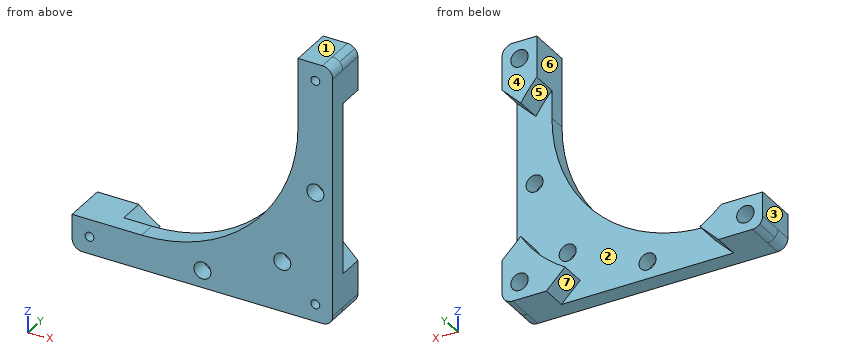
```python
from build123d import *

# Parameters (mm, degrees)
SKETCH1_W               = 190.5
SKETCH1_H               = 190.5
BOSS_EXTRUDE1_DEPTH     = 12.7
FILLET1_R               = 7.62
BOSS_EXTRUDE3_START     = 19.05
BOSS_EXTRUDE3_DEPTH     = 19.05
CIRPATTERN1_COUNT       = 4
SKETCH8_R               = 6.223
CUT_EXTRUDE2_DEPTH      = 25.4
CUT_EXTRUDE3_DEPTH      = 137.044211564
CUT_EXTRUDE3_DEPTH_BACK = 137.044211564
SKETCH10_R              = 6.223
FILLET2_R               = 12.7
SKETCH11_R              = 6.35
CUT_EXTRUDE4_DEPTH      = 19.05
SKETCH11_3_R            = 3.2385
CUT_EXTRUDE5_DEPTH      = 139.395041457
CIRPATTERN2_COUNT       = 4
CUT_EXTRUDE6_DEPTH      = 137.044211564
CUT_EXTRUDE6_DEPTH_BACK = 137.044211564
CUT_EXTRUDE7_DEPTH      = 137.044211564
CUT_EXTRUDE7_DEPTH_BACK = 137.044211564


with BuildPart() as part:
    # Sketch1 → Boss-Extrude1 (new body)
    with BuildSketch(Plane(origin=(0, 0, 0), x_dir=(1, 0, 0), z_dir=(0, 1, 0))):
        Rectangle(SKETCH1_W, SKETCH1_H)
    extrude(amount=BOSS_EXTRUDE1_DEPTH)

    # Fillet1
    fillet1_edges = [part.edges().sort_by_distance(p)[0] for p in [
        (95.25, 6.35, 95.25),
        (-95.25, 6.35, 95.25),
        (-95.25, 6.35, -95.25),
        (95.25, 6.35, -95.25),
    ]]
    fillet(fillet1_edges, radius=FILLET1_R)

    # Sketch7 → Boss-Extrude3 (add)
    with BuildSketch(Plane(origin=(0, 12.7, 0), x_dir=(1, 0, 0), z_dir=(0, 1, 0)).offset(BOSS_EXTRUDE3_START)):
        with BuildLine():
            Line((67.396822189, 67.396822189), (93.018153673, 93.018153673))
            ThreePointArc((93.018153673, 93.018153673), (90.546047755, 94.669962038), (87.63, 95.25))
            Line((87.63, 95.25), (62.921077964, 95.25))
            Line((62.921077964, 95.25), (49.265209936, 81.594131972))
            ThreePointArc((49.265209936, 81.594131972), (58.761367718, 75.045086089), (67.396822189, 67.396822189))
        make_face()
        with BuildLine():
            ThreePointArc((95.25, 87.63), (94.669962038, 90.546047755), (93.018153673, 93.018153673))
            Line((93.018153673, 93.018153673), (67.396822189, 67.396822189))
            ThreePointArc((67.396822189, 67.396822189), (75.045086089, 58.761367718), (81.594131972, 49.265209936))
            Line((81.594131972, 49.265209936), (95.25, 62.921077964))
            Line((95.25, 62.921077964), (95.25, 87.63))
        make_face()
    boss_extrude3 = extrude(amount=-BOSS_EXTRUDE3_DEPTH)

    # CirPattern1: Boss-Extrude3 ×4 about axis
    cirpattern1_axis = Axis((0, 0, 0), (0, 1, 0))
    for i in range(1, CIRPATTERN1_COUNT):
        add(boss_extrude3.rotate(cirpattern1_axis, i * 360 / CIRPATTERN1_COUNT))

    # Sketch8 → Cut-Extrude2 (cut)
    with BuildSketch(Plane(origin=(0, 12.7, 0), x_dir=(1, 0, 0), z_dir=(0, 1, 0))):
        with Locations(Location((0, 82.55, 0), (0, 0, 270))):
            Circle(SKETCH8_R)
        with Locations(Location((58.371664787, 58.371664787, 0), (0, 0, 270))):
            Circle(SKETCH8_R)
        with Locations(Location((82.55, 0, 0), (0, 0, 270))):
            Circle(SKETCH8_R)
        with Locations(Location((58.371664787, -58.371664787, 0), (0, 0, 270))):
            Circle(SKETCH8_R)
        with Locations(Location((0, -82.55, 0), (0, 0, 270))):
            Circle(SKETCH8_R)
        with Locations(Location((-58.371664787, -58.371664787, 0), (0, 0, 270))):
            Circle(SKETCH8_R)
        with Locations(Location((-82.55, 0, 0), (0, 0, 270))):
            Circle(SKETCH8_R)
        with Locations(Location((-58.371664787, 58.371664787, 0), (0, 0, 270))):
            Circle(SKETCH8_R)
    extrude(amount=-CUT_EXTRUDE2_DEPTH, mode=Mode.SUBTRACT)

    # Sketch10 → Cut-Extrude3 (cut, two sides: drawn at the far end of the back side and taken through both)
    # profile 1 of 2: a face of its own
    with BuildSketch(Plane(origin=(0, 12.7, 0), x_dir=(1, 0, 0), z_dir=(0, 1, 0)).offset(-CUT_EXTRUDE3_DEPTH_BACK)):
        Polygon((38.1, 38.1), (-95.25, 38.1), (-95.25, -38.1), (-38.1, -38.1), (-38.1, -95.25), (38.1, -95.25), align=None)
        with Locations((-82.55, 0)):
            Circle(SKETCH10_R, mode=Mode.SUBTRACT)
        with Locations((0, -82.55)):
            Circle(SKETCH10_R, mode=Mode.SUBTRACT)
    # profile 2 of 2: a face of its own
    with BuildSketch(Plane(origin=(0, 12.7, 0), x_dir=(1, 0, 0), z_dir=(0, 1, 0)).offset(-CUT_EXTRUDE3_DEPTH_BACK)):
        with BuildLine():
            Line((-38.1, -38.1), (-95.25, -38.1))
            Line((-95.25, -38.1), (-95.25, -62.921077964))
            Line((-95.25, -62.921077964), (-81.594131972, -49.265209936))
            ThreePointArc((-81.594131972, -49.265209936), (-67.396822189, -67.396822189), (-49.265209936, -81.594131972))
            Line((-49.265209936, -81.594131972), (-62.921077964, -95.25))
            Line((-62.921077964, -95.25), (-38.1, -95.25))
            Line((-38.1, -95.25), (-38.1, -38.1))
        make_face()
        with Locations((-58.371664787, -58.371664787)):
            Circle(SKETCH10_R, mode=Mode.SUBTRACT)
    extrude(amount=CUT_EXTRUDE3_DEPTH + CUT_EXTRUDE3_DEPTH_BACK, mode=Mode.SUBTRACT)


with BuildPart() as cut_extrude3_kept_piece:
    # of the separate pieces the step leaves, the one the design keeps (cut_extrude3_pieces_kept)
    add(part.part.solids().sort_by_distance((38.1, 0, 95.25))[0])

    # Fillet2
    fillet2_edges = [cut_extrude3_kept_piece.edges().sort_by_distance(p)[0] for p in [
        (-95.25, 6.35, -38.1),
        (38.1, 6.35, -38.1),
        (38.1, 6.35, 95.25),
    ]]
    fillet(fillet2_edges, radius=FILLET2_R)

    # Sketch11 → Cut-Extrude4 (cut)
    with BuildSketch(Plane(origin=(0, 31.75, 0), x_dir=(1, 0, 0), z_dir=(0, 1, 0))):
        with Locations(Location((82.55, 82.55, 0), (0, 0, 270))):
            Circle(SKETCH11_R)
    cut_extrude4 = extrude(amount=-CUT_EXTRUDE4_DEPTH, mode=Mode.SUBTRACT)

    # Sketch11<3> → Cut-Extrude5 (cut, through all)
    with BuildSketch(Plane(origin=(0, 31.75, 0), x_dir=(1, 0, 0), z_dir=(0, 1, 0))):
        with Locations(Location((82.55, 82.55, 0), (0, 0, 270))):
            Circle(SKETCH11_3_R)
    cut_extrude5 = extrude(amount=-CUT_EXTRUDE5_DEPTH, mode=Mode.SUBTRACT)

    # CirPattern2: Cut-Extrude4, Cut-Extrude5 ×4 about axis
    cirpattern2_axis = Axis((0, 0, 0), (0, 1, 0))
    add([cut_extrude4.rotate(cirpattern2_axis, i * 360 / CIRPATTERN2_COUNT) for i in range(1, CIRPATTERN2_COUNT)], mode=Mode.SUBTRACT)
    add([cut_extrude5.rotate(cirpattern2_axis, i * 360 / CIRPATTERN2_COUNT) for i in range(1, CIRPATTERN2_COUNT)], mode=Mode.SUBTRACT)

    # Sketch12 → Cut-Extrude6 (cut, two sides: drawn at the far end of the back side and taken through both)
    with BuildSketch(Plane(origin=(0, 12.7, 0), x_dir=(1, 0, 0), z_dir=(0, 1, 0)).offset(-CUT_EXTRUDE6_DEPTH_BACK)):
        Polygon((-95.25, -95.25), (69.85, -95.25), (69.85, -44.45), (-44.45, -44.45), (-44.45, 69.85), (-95.25, 69.85), align=None)
    extrude(amount=CUT_EXTRUDE6_DEPTH + CUT_EXTRUDE6_DEPTH_BACK, mode=Mode.SUBTRACT)

    # Sketch13 → Cut-Extrude7 (cut, two sides: drawn at the far end of the back side and taken through both)
    with BuildSketch(Plane(origin=(0, 12.7, 0), x_dir=(1, 0, 0), z_dir=(0, 1, 0)).offset(-CUT_EXTRUDE7_DEPTH_BACK)):
        with BuildLine():
            Line((-44.45, 69.85), (-44.45, -44.45))
            Line((-44.45, -44.45), (69.85, -44.45))
            ThreePointArc((69.85, -44.45), (36.37230509, 36.37230509), (-44.45, 69.85))
        make_face()
    extrude(amount=CUT_EXTRUDE7_DEPTH + CUT_EXTRUDE7_DEPTH_BACK, mode=Mode.SUBTRACT)


solid = cut_extrude3_kept_piece.part
```
For this review, take the finished solid that the model builds, in its own axes (mm). Face numbers are marked on the shaded views. A direction names the side the tool comes from. Give positions to 0.01 mm unless a question says otherwise; leave off trailing zeros. Order: outer loops, then holes, each group sorted by start corner. A loop starts at its lowest first (then second) coordinate and runs counter-clockwise, first axis right, second up.
1) Take a section at D-D (x = 0). Give the boundary of the cut face in (y, z).
2) Wall thickness on line 1 (Z direction, x = 82, y = 6); line 2 (X direction, y = 25, z = -83.5); line 3 (Y direction, x = 83.5, z = -18.5): over which ranges is each line inside the solid? List them lowest first.
3) Insertion check: pin 1 (8.5 mm diameter, centred on x = -82.55, z = -82.55, fed in from +Y); pin 2 (12 mm diameter, centred on y = 26, z = 65, fed in from -X); pin 3 (9.5 mm diameter, centred on y = 20, z = 80, fed in from -X). Each pin has a flat end and moves straight along its axis. Give the tip position at first contact, or say it passes through.
4) For the marked faces 4, 5, 6 and 7, list the 3-axis set-ups (+Z, -Z, +X, -X, +Y, -Y) from which the entire face can be reached by the end or side of a thin tool; tool diameter is ignored.
5) Take a section at B-B (z = 82.55). Give the boundary of the cut face in (x, y), then the cut area to 3 significant figures.
6) The part is to be moulded in two halves that separate along Z. For the marked faces 1, 2 and 3, say which applies: released by +Z, released by -Z, zero draft, split by the parting line, or undercut.
7) Take a section at C-C (x = -82.5). Give the boundary of the cut face in (y, z).
8) Take a section at A-A (y = 15.5). Give the boundary of the cut face in (x, z).
Derived:
1. outline: (0, -95.25) - (12.7, -95.25) - (12.7, -88.77) - (0, -88.77) - close; (0, -76.33) - (12.7, -76.33) - (12.7, -60.85) - (0, -60.85) - close
2. line 1: z = -95.25 to -85.74, -79.36 to -6.2, 6.2 to 79.36, 85.74 to 95.25
2. line 2: x = -95.25 to -88.83, -76.27 to -51.17, 51.17 to 76.27, 88.83 to 95.25
2. line 3: y = 0 to 12.7
3. pin 1: stops at y = 12.7
3. pin 2: stops at x = 69.85
3. pin 3: stops at x = 69.85
4. face 4: +Z, -Z, +X, -X, +Y
4. face 5: -X, +Y
4. face 6: +Z, -X, +Y, -Y
4. face 7: -Z, +Y
5. outline: (69.85, 0) - (79.31, 0) - (79.31, 12.7) - (76.2, 12.7) - (76.2, 31.75) - (69.85, 31.75) - close; (85.79, 0) - (95.25, 0) - (95.25, 31.75) - (88.9, 31.75) - (88.9, 12.7) - (85.79, 12.7) - close
5. area: 482 mm2
6. face 1: released by +Z
6. face 2: undercut
6. face 3: zero draft
7. outline: (0, -95.25) - (31.75, -95.25) - (31.75, -88.9) - (12.7, -88.9) - (12.7, -85.79) - (0, -85.79) - close; (0, -79.31) - (12.7, -79.31) - (12.7, -76.2) - (31.75, -76.2) - (31.75, -69.85) - (0, -69.85) - close
8. outline: (-95.25, -87.63) arc R7.62 ccw to (-87.63, -95.25) - (-62.92, -95.25) - (-49.27, -81.59) arc R95.31 cw to (-64.85, -69.85) - (-95.25, -69.85) - close; (49.27, -81.59) - (62.92, -95.25) - (87.63, -95.25) arc R7.62 ccw to (95.25, -87.63) - (95.25, -62.92) - (81.59, -49.27) arc R95.31 cw to start; (69.85, 64.85) arc R95.31 cw to (81.59, 49.27) - (95.25, 62.92) - (95.25, 87.63) arc R7.62 ccw to (87.63, 95.25) - (69.85, 95.25) - close; hole circle Ø12.7 at (-82.55, -82.55); hole circle Ø12.7 at (82.55, -82.55); hole circle Ø12.7 at (82.55, 82.55)
